```python
from build123d import *

# Parameters (mm, degrees)
F1_DEPTH = 20
F2_R     = 6
F3_DEPTH = 25
F5_DEPTH = 12


with BuildPart() as f1:
    # F0 (on Top) → F1 (new body)
    with BuildSketch(Plane.XY):
        with BuildLine():
            ThreePointArc((90, 30), (84.142136, 44.142136), (70, 50))
            Line((70, 50), (-70, 50))
            ThreePointArc((-70, 50), (-84.142136, 44.142136), (-90, 30))
            Line((-90, 30), (-90, -30))
            ThreePointArc((-90, -30), (-84.142136, -44.142136), (-70, -50))
            Line((-70, -50), (70, -50))
            ThreePointArc((70, -50), (84.142136, -44.142136), (90, -30))
            Line((90, -30), (90, 30))
        make_face()
    extrude(amount=-F1_DEPTH)

    # F2 (on face) → F3 (cut)
    with BuildSketch(Plane.XY):
        with Locations((70, 30)):
            Circle(F2_R)
        with Locations((-70, 30)):
            Circle(F2_R)
        with Locations((70, -30)):
            Circle(F2_R)
        with Locations((-70, -30)):
            Circle(F2_R)
    extrude(amount=-F3_DEPTH, mode=Mode.SUBTRACT)

    # F4 (on face) → F5 (cut)
    with BuildSketch(Plane.XY):
        with BuildLine():
            Line((27.658633, -10), (32, -10))
            ThreePointArc((32, -10), (37.656854, -7.656854), (40, -2))
            Line((40, -2), (40, 2))
            ThreePointArc((40, 2), (37.656854, 7.656854), (32, 10))
            Line((32, 10), (27.658633, 10))
            ThreePointArc((27.658633, 10), (23.844783, 10.967607), (20.95351, 13.636364))
            ThreePointArc((20.95351, 13.636364), (0, 25), (-20.95351, 13.636364))
            ThreePointArc((-20.95351, 13.636364), (-23.844783, 10.967607), (-27.658633, 10))
            Line((-27.658633, 10), (-32, 10))
            ThreePointArc((-32, 10), (-37.656854, 7.656854), (-40, 2))
            Line((-40, 2), (-40, -2))
            ThreePointArc((-40, -2), (-37.656854, -7.656854), (-32, -10))
            Line((-32, -10), (-27.658633, -10))
            ThreePointArc((-27.658633, -10), (-23.844783, -10.967607), (-20.95351, -13.636364))
            ThreePointArc((-20.95351, -13.636364), (0, -25), (20.95351, -13.636364))
            ThreePointArc((20.95351, -13.636364), (23.844783, -10.967607), (27.658633, -10))
        make_face()
    extrude(amount=-F5_DEPTH, mode=Mode.SUBTRACT)


solid = f1.part
```
Work out the finished part from the listing and answer in its coordinate system (mm). A direction names the side the tool comes from. Give positions to 0.01 mm unless a question says otherwise; leave off trailing zeros. Loops run counter-clockwise (first coordinate to the right, second up) from the corner with the lowest first, then second, coordinate; pieces in that order, holes last. Notation, with made-up numbers: (32.25, 82.25) - (77.25, 82.25) arc R20 ccw to (77.25, 89.25) - close; hole circle Ø11 at (-12.5, -21.75). An arc over 180 degrees is marked (long way). One line per question, with ' | ' between items.
(1) Each of these flat-tipped pins is pushed along its axis until it touches: pin 1 Ø25 at (x, y) = (-13, -11.5) entering from +Z; pin 2 Ø1 at (y, z) = (32, -3) entering from +X; pin 3 Ø11 at (x, y) = (-70, 30) entering from +Z. Where does it stop, or does it pass through?
Recorded:
pin 1: stops at z = 0 | pin 2: stops at x = 89.94 | pin 3: passes through
(2) Straight lines are drawn through the part: probe 1 along Y at (x, z) = (-70, -6.5); probe 2 along X at (y, z) = (-26, -11.5); probe 3 along Y at (x, z) = (-73.5, -13). For each, find the intervals that lie inside material, in ascending order.
Recorded:
probe 1: y = -50 to -36, -24 to 24, 36 to 50 | probe 2: x = -90 to -74.47, -65.53 to 65.53, 74.47 to 90 | probe 3: y = -49.69 to -34.87, -25.13 to 25.13, 34.87 to 49.69
(3) The part is cut by section B-B (y = 33.5). Write down the section's boundary in (x, z).
Recorded:
outline: (-89.69, -20) - (-74.87, -20) - (-74.87, 0) - (-89.69, 0) - close; (-65.13, -20) - (65.13, -20) - (65.13, 0) - (-65.13, 0) - close; (74.87, -20) - (89.69, -20) - (89.69, 0) - (74.87, 0) - close
(4) The part is cut by section A-A (z = -5.5). Write down the section's boundary in (x, y).
Recorded:
outline: (-90, -30) arc R20 ccw to (-70, -50) - (70, -50) arc R20 ccw to (90, -30) - (90, 30) arc R20 ccw to (70, 50) - (-70, 50) arc R20 ccw to (-90, 30) - close; hole circle Ø12 at (-70, -30); hole circle Ø12 at (-70, 30); hole (-40, -2) arc R8 ccw to (-32, -10) - (-27.66, -10) arc R8 cw to (-20.95, -13.64) arc R25 ccw to (20.95, -13.64) arc R8 cw to (27.66, -10) - (32, -10) arc R8 ccw to (40, -2) - (40, 2) arc R8 ccw to (32, 10) - (27.66, 10) arc R8 cw to (20.95, 13.64) arc R25 ccw to (-20.95, 13.64) arc R8 cw to (-27.66, 10) - (-32, 10) arc R8 ccw to (-40, 2) - close; hole circle Ø12 at (70, -30); hole circle Ø12 at (70, 30)
(5) The mould has two halves that part along X. Classify faces 1 (the face through (37.719, 7.594, -5.916)), 2 (the face through (83.986, -44.297, -9.86)), 3 (the face through (-1, 1, -20)): +X half, -X half, draft (parallel to the pull), parting line (faces both ways), or undercut.
Recorded:
face 1: undercut | face 2: +X half | face 3: draft
(6) The part is cut by section C-C (z = -17.5). Write down the section's boundary in (x, y), then the cut area to 3 significant figures.
Recorded:
outline: (-90, -30) arc R20 ccw to (-70, -50) - (70, -50) arc R20 ccw to (90, -30) - (90, 30) arc R20 ccw to (70, 50) - (-70, 50) arc R20 ccw to (-90, 30) - close; hole circle Ø12 at (-70, -30); hole circle Ø12 at (-70, 30); hole circle Ø12 at (70, -30); hole circle Ø12 at (70, 30) | area: 17,200 mm²
(7) A tool of negligible diameter and unlimited length cuts with its end or side. For faces 4 (the face through (84.297, 43.986, -9.86)), 5 (the face through (30, 10, -6)), from which of +Z, -Z, +X, -X, +Y, -Y can it reach the whole face along a straight path? Write none if from no direction.
Recorded:
face 4: +Z, -Z, +X, +Y | face 5: +Z
(8) The part is cut by section D-D (y = -21). Write down the section's boundary in (x, z), then the cut area to 3 significant figures.
Recorded:
outline: (-90, -20) - (90, -20) - (90, 0) - (13.56, 0) - (13.56, -12) - (-13.56, -12) - (-13.56, 0) - (-90, 0) - close | area: 3,270 mm²
